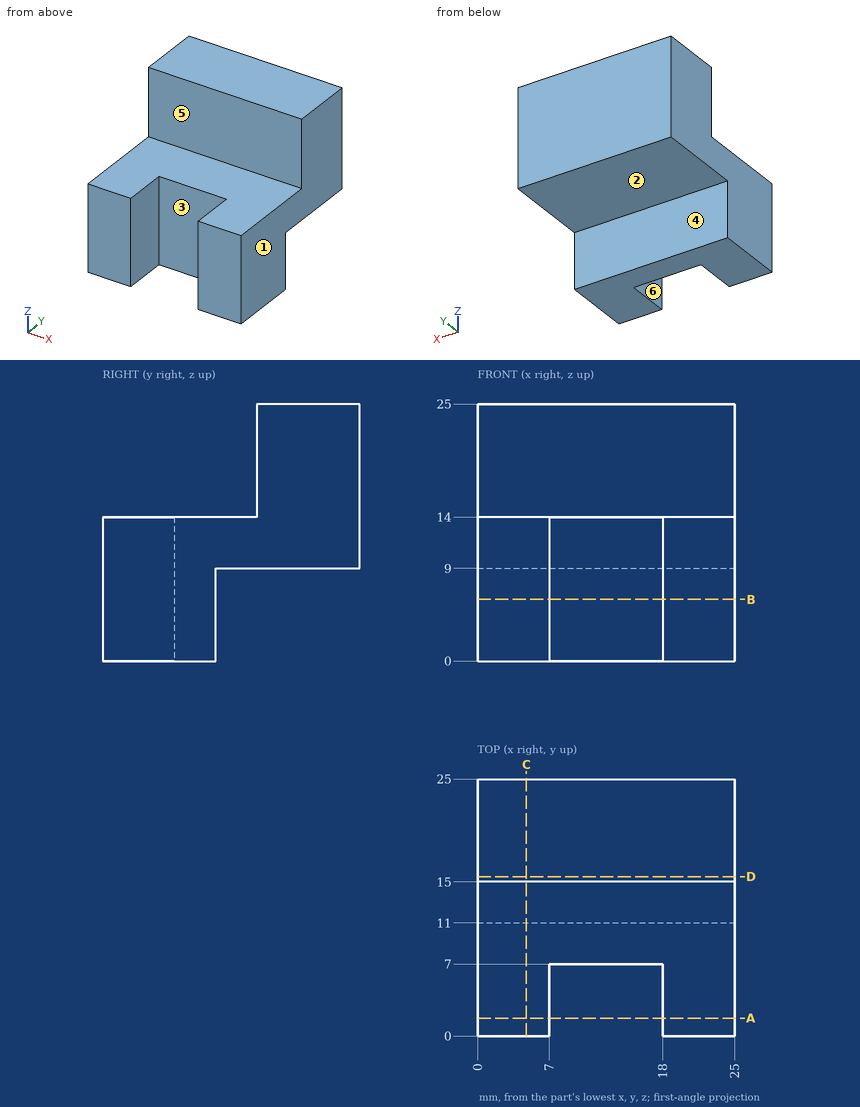
Study the drawing (mm; zero at the part's minimum x, y, z) and answer. A direction names the side the tool comes from. Give positions to 0.01 mm unless a question says otherwise; leave off trailing zeros. Order: outer loops, then holes, each group sorted by start corner. A loop starts at its lowest first (then second) coordinate and runs counter-clockwise, first axis right, second up.
1. Section B-B, the plane z = 6 is taken. Determine the outline of the cut face in (x, y).
Result sheet:
outline: (0, 0) - (7, 0) - (7, 7) - (18, 7) - (18, 0) - (25, 0) - (25, 11) - (0, 11) - close
2. Section A-A, the plane y = 1.75 is taken. Determine the outline of the cut face in (x, z), and give its area (3 significant figures).
Result sheet:
outline: (0, 0) - (7, 0) - (7, 14) - (0, 14) - close; (18, 0) - (25, 0) - (25, 14) - (18, 14) - close
area: 196 mm2
3. Straight lines are drawn through the part: L1, parallel to X at y = 5, z = 7; L2, parallel to Z at x = 18.75, y = 17.75; L3, parallel to Z at x = 2, y = 8. For each, find the intervals that lie inside material, in ascending order.
Result sheet:
L1: x = 0 to 7, 18 to 25
L2: z = 9 to 25
L3: z = 0 to 14
4. Section D-D, the plane y = 15.5 is taken. Determine the outline of the cut face in (x, z), and give its area (3 significant figures).
Result sheet:
outline: (0, 9) - (25, 9) - (25, 25) - (0, 25) - close
area: 400 mm2
5. Section C-C, the plane x = 4.75 is taken. Determine the outline of the cut face in (y, z), and give its area (3 significant figures).
Result sheet:
outline: (0, 0) - (11, 0) - (11, 9) - (25, 9) - (25, 25) - (15, 25) - (15, 14) - (0, 14) - close
area: 334 mm2
6. For the marked faces 4, 5 and 6, determine the directions among +Z, -Z, +X, -X, +Y, -Y from which every point of the face is accessible in a straight line to the end or side of a thin tool.
Result sheet:
face 4: -Z, +X, -X, +Y
face 5: +Z, +X, -X, -Y
face 6: +Z, -Z, -Y
7. The mould has two halves that part along X. Classify the marked faces 1, 2 and 3: released by +X, released by -X, zero draft, split by the parting line, or undercut.
Result sheet:
face 1: released by +X
face 2: zero draft
face 3: undercut
8. Each of these flat-tipped pins is pushed along its axis until it touches: P1, Ø6, axis at y = 9, z = 11, coming from the -X side; P2, Ø9, axis at x = 15, z = 20.5, coming from the -Y side; P3, Ø2.5, axis at x = 6.5, z = 5, coming from the +Y side; P4, Ø9, axis at x = 13, z = 4.5, coming from the -Y side. Where does it stop, or does it pass through?
Result sheet:
P1: stops at x = 0
P2: stops at y = 15
P3: stops at y = 11
P4: stops at y = 7
